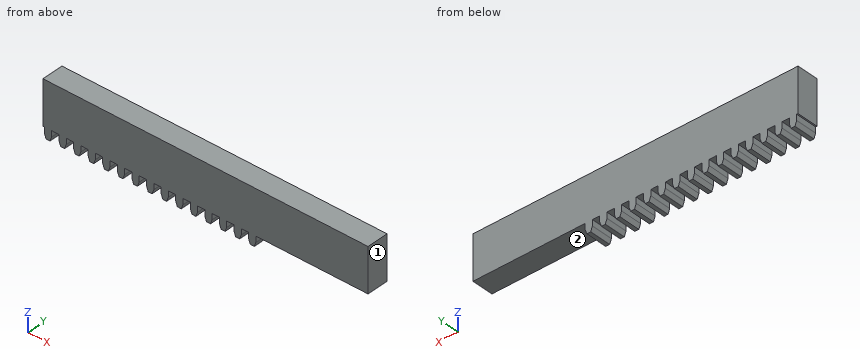
from build123d import *

# Parameters (mm, degrees)
SKETCH2_W           = 130
SKETCH2_H           = 19
BOSS_EXTRUDE1_DEPTH = 9.3
BOSS_EXTRUDE2_DEPTH = 9.3
LPATTERN1_COUNT     = 11
LPATTERN1_PITCH     = 6.283185307
LPATTERN1_COL_COUNT = 5
LPATTERN1_COL_PITCH = 6.283185307
SKETCH3_W           = 19
SKETCH3_H           = 9.3
BOSS_EXTRUDE3_DEPTH = 10


with BuildPart() as part:
    # Sketch2 → Boss-Extrude1 (new body)
    with BuildSketch(Plane(origin=(0, 0, 0), x_dir=(1, 0, 0), z_dir=(0, 1, 0))):
        with Locations((0, -9.5)):
            Rectangle(SKETCH2_W, SKETCH2_H)
    extrude(amount=BOSS_EXTRUDE1_DEPTH)

    # Sketch2<5> → Boss-Extrude2 (add)
    with BuildSketch(Plane(origin=(0, 0, 0), x_dir=(1, 0, 0), z_dir=(0, 1, 0))):
        Polygon((0.842855858, 4.499999971), (-0.842855858, 4.499999971), (-1.571175787, 2.500138124), (-1.571175787, 0), (1.570796327, 0), (1.570796327, 2.499999971), align=None)
    boss_extrude2 = extrude(amount=BOSS_EXTRUDE2_DEPTH)

    # LPattern1: Boss-Extrude2 ×11
    with Locations(*[(-i * LPATTERN1_PITCH, 0, 0) for i in range(1, LPATTERN1_COUNT)]):
        add(boss_extrude2)

    # LPattern1 col: Boss-Extrude2 ×5
    with Locations(*[(i * LPATTERN1_COL_PITCH, 0, 0) for i in range(1, LPATTERN1_COL_COUNT)]):
        add(boss_extrude2)

    # Sketch3 → Boss-Extrude3 (add)
    with BuildSketch(Plane(origin=(65, 0, 0), x_dir=(0, 0, -1), z_dir=(1, 0, 0))):
        with Locations((-9.5, 4.65)):
            Rectangle(SKETCH3_W, SKETCH3_H)
    extrude(amount=BOSS_EXTRUDE3_DEPTH)


solid = part.part
Read the model definition and answer for the solid it produces. Units are mm, in the model's axes. Face numbers are marked on the shaded views. A direction names the side the tool comes from. Coordinates: 2 decimals unless noted, no trailing zeros. Order: outer loops, then holes, each group sorted by start corner. A loop starts at its lowest first (then second) coordinate and runs counter-clockwise, first axis right, second up. Notation, with made-up numbers: M 1.25,3.25 L 50.25,3.25 A25 ccw 50.25,35.25 Z; hole C 86.25,7.5 d6. An arc over 180 degrees is marked long. Put each result on its own line as item: value. Start each with the question number.
Item 1: For the marked faces 1 and 2, determine the directions among +Z, -Z, +X, -X, +Y, -Y from which every point of the face is accessible in a straight line to the end or side of a thin tool.
Item 2: Section A-A, the plane x = 31.5 is taken. Determine the outline of the cut face in (y, z).
Item 3: Given pin 1 Ø1.2 at (y, z) = (3.5, -1) entering from +X; pin 2 Ø1.3 at (y, z) = (6.5, -1.5) entering from -X; pin 3 Ø4 at (x, y) = (50.5, 4.5) entering from -Z; pin 4 Ø3.5 at (x, y) = (-41.5, 7) entering from -Z, each flat-ended and moving along its own axis, determine where each tip first touches the part or whether it passes through.
Item 4: Consider probe 1 along Z at (x, y) = (60.5, 6). Determine where the line is inside the solid, lowest interval first. Write a range as [from, to].
Computed:
1. face 1: +Z, -Z, +X, +Y, -Y
1. face 2: -Z, +X, +Y, -Y
2. outline: M 0,0 L 9.3,0 L 9.3,19 L 0,19 Z
3. pin 1: stops at x = 26.7
3. pin 2: stops at x = -64.4
3. pin 3: stops at z = 0
3. pin 4: stops at z = -4.5
4. probe 1: z = [0, 19]
